Geometry: final body of the model. Coordinates: model frame, mm. Give positions to 0.01 mm unless a question says otherwise; leave off trailing zeros. Write each loop counter-clockwise with the first axis right and the second up, starting at its lowest first coordinate (ties: lowest second). Pieces come first, ordered by that corner, then holes.
Q1. Line query: L1, parallel to Y at x = 0, z = 3.3; L2, parallel to X at y = 2.25, z = 1.3; L3, parallel to X at y = 1.25, z = 1.85. Output: solid intervals per line, ascending.
Q2. Cut plane D-D on z = 4.4. Return the cut outline in (x, y), plus the area to 3 significant figures.
Q3. Cut plane A-A on x = 0. Return the cut outline in (y, z).
Q4. Cut plane C-C on z = 3.45. Return the cut outline in (x, y), plus the area to 3 significant figures.
```python
from build123d import *

# Parameters (mm, degrees)
SKETCH_W    = 10
SKETCH_H    = 10
SKETCH_R    = 3.2
PAD_DEPTH   = 5
FILLET_R    = 1
FILLET001_R = 1


with BuildPart() as part:
    # Sketch → Pad (new body)
    with BuildSketch(Plane.XY):
        Rectangle(SKETCH_W, SKETCH_H)
        Circle(SKETCH_R, mode=Mode.SUBTRACT)
    extrude(amount=PAD_DEPTH)

    # Fillet
    fillet_edges = [part.edges().sort_by_distance(p)[0] for p in [
        (-3.2, 0, 0),
    ]]
    fillet(fillet_edges, radius=FILLET_R)

    # Fillet001
    fillet001_edges = [part.edges().sort_by_distance(p)[0] for p in [
        (-3.2, 0, 5),
    ]]
    fillet(fillet001_edges, radius=FILLET001_R)


solid = part.part
```
Data:
1. L1: y = -5 to -3.2, 3.2 to 5
1. L2: x = -5 to -2.28, 2.28 to 5
1. L3: x = -5 to -2.95, 2.95 to 5
2. outline: (-5, -5) - (5, -5) - (5, 5) - (-5, 5) - close; hole circle Ø6.57 at (0, 0)
2. area: 66.1 mm2
3. outline: (-5, 0) - (-4.2, 0) arc R1 ccw to (-3.2, 1) - (-3.2, 4) arc R1 ccw to (-4.2, 5) - (-5, 5) - close; (3.2, 1) arc R1 ccw to (4.2, 0) - (5, 0) - (5, 5) - (4.2, 5) arc R1 ccw to (3.2, 4) - close
4. outline: (-5, -5) - (5, -5) - (5, 5) - (-5, 5) - close; hole circle Ø6.4 at (0, 0)
4. area: 67.8 mm2
